Can you work these out from the model? Positions are in its coordinate system, mm. Round coordinates to 2 decimals unless told otherwise and drop trailing zeros. Order: outer loops, then holes, each group sorted by start corner. A loop starts at its lowest first (then second) coordinate and runs counter-clockwise, first axis right, second up. Notation, with made-up numbers: (43, 5) -> (94, 5) arc R22 cw to (94, 38) -> close; hole circle Ø7 at (40, 42.25). An arc over 180 degrees is marked (long way). Use a Markdown table: item, result. Add a question column.
Q1. We'd pull the mould along Z, two halves only. Please class faces 1 (the face through (0, 0, 660.4)), 2 (the face through (0, 0, 0)), 3 (the face through (-1.379, 12.626, 647.441)): +Z half, -Z half, draft (parallel to the pull), parting line (faces both ways), or undercut.
Q2. I'm going to push flat-ended pins straight in: pin 1 Ø10 at (x, z) = (5, 185.5) entering from +Y; pin 2 Ø4 at (y, z) = (-8, 454) entering from +X; pin 3 Ø5 at (x, z) = (7.5, 583.5) entering from -Y; pin 4 Ø12 at (y, z) = (4, 566.5) entering from +X. Where does each tip first touch, or does it pass through?
Q3. If we section it at A-A on z = 246: List the corners of the cut face in (x, y) for me, plus the area to 3 significant figures.
Q4. I need wall thicknesses on line 1 along Z through (x, y) = (1.25, -11.25); line 2 along Z through (x, y) = (0, 12); line 3 along Y through (x, z) = (0.5, 111). Which ranges of each line are inside material? Lowest first, please. Write a range as [from, to].
```python
from build123d import *

# Parameters (mm, degrees)
BOSS_EXTRUDE1_DEPTH = 660.4
SKETCH2_RX          = 7.33298
SKETCH2_RY          = 7.27642549
CUT_EXTRUDE1_DEPTH  = 33.02


with BuildPart() as part:
    # Sketch1 → Boss-Extrude1 (new body)
    with BuildSketch(Plane.XY):
        Polygon((5.802204234, 13.469402687), (-8.763742784, 11.759557608), (-14.565947018, -1.709845079), (-5.802204234, -13.469402687), (8.763742784, -11.759557608), (14.565947018, 1.709845079), align=None)
    extrude(amount=BOSS_EXTRUDE1_DEPTH)

    # Sketch2 → Cut-Extrude1 (cut)
    with BuildSketch(Plane(origin=(-1.480769275, 12.614480148, 0), x_dir=(0.9931806044692795, 0.11658596358926146, 0), z_dir=(-0.11658596358926147, 0.9931806044692796, 0))):
        with Locations(Location((0, -627.66702), (0, 0, 180))):
            Ellipse(SKETCH2_RX, SKETCH2_RY)
    extrude(amount=-CUT_EXTRUDE1_DEPTH, mode=Mode.SUBTRACT)


solid = part.part
```
Answer below:
| question | item | result |
|---|---|---|
| 1 | face 1 | +Z half |
| 1 | face 2 | -Z half |
| 1 | face 3 | draft |
| 2 | pin 1 | y = 13.47 |
| 2 | pin 2 | x = 11.24 |
| 2 | pin 3 | y = -12.2 |
| 2 | pin 4 | x = 14.57 |
| 3 | outline | (-14.57, -1.71) -> (-5.8, -13.47) -> (8.76, -11.76) -> (14.57, 1.71) -> (5.8, 13.47) -> (-8.76, 11.76) -> close |
| 3 | area | 559 mm² |
| 4 | line 1 | [0, 620.39], [634.94, 660.4] |
| 4 | line 2 | [0, 620.52], [634.81, 660.4] |
| 4 | line 3 | [-12.73, 12.85] |
